```python
from build123d import *

# Parameters (mm, degrees)
F0_R     = 4
F0_R_2   = 5
F1_DEPTH = 8.5


with BuildPart() as f1:
    # F0 (on Top) → F1 (new body, symmetric)
    with BuildSketch(Plane.XY):
        with BuildLine():
            ThreePointArc((175, -20), (195, 0), (175, 20))
            Line((175, 20), (-175, 20))
            ThreePointArc((-175, 20), (-195, 0), (-175, -20))
            Line((-175, -20), (175, -20))
        make_face()
        with Locations((-175, 0)):
            Circle(F0_R, mode=Mode.SUBTRACT)
        Circle(F0_R_2, mode=Mode.SUBTRACT)
        with Locations((175, 0)):
            Circle(F0_R, mode=Mode.SUBTRACT)
    extrude(amount=F1_DEPTH, both=True)


solid = f1.part
```
Geometry: final body of the model. Coordinates: model frame, mm. Round coordinates to 2 decimals unless told otherwise and drop trailing zeros. Write each loop counter-clockwise with the first axis right and the second up, starting at its lowest first coordinate (ties: lowest second). Pieces come first, ordered by that corner, then holes. Notation, with made-up numbers: M 29,15.25 L 71,15.25 A15 cw 71,35.25 Z; hole C -35,61.5 d11. An arc over 180 degrees is marked long. Answer in a Markdown table with one row per item. Add a question column.
(1) Ray query, L1, parallel to Y at x = 175, z = -0.25; L2, parallel to X at y = 3, z = 1.5; L3, parallel to X at y = -1, z = 1.5. Return the intervals inside material, ascending.
(2) Cut plane B-B, the plane z = 5.25. Return the cut outline in (x, y), then the cut area to 3 significant figures.
(3) Cut plane C-C, the plane y = 0. Return the cut outline in (x, z), then the cut area to 3 significant figures.
(4) Cut plane A-A, the plane x = 0. Return the cut outline in (y, z), then the cut area to 3 significant figures.
(5) Draft query along Y for faces 1 (the face through (195, 0, 0)), 2 (the face through (-3, 5, -8.5)), 3 (the face through (178.815, 1.201, -0.119)). Return one class per face: pulls with the +Y half, pulls with the -Y half, needs draft (parallel to the pull), parting line crosses it, or undercut.
(6) Cut plane D-D, the plane y = -15.5. Return the cut outline in (x, z), then the cut area to 3 significant figures.
(7) Contact query for flat-ended pins moving along their axis: pin 1 (5 mm diameter, centred on y = -4, z = -3, fed in from -X); pin 2 (5 mm diameter, centred on y = 1, z = -2, fed in from -X); pin 3 (2 mm diameter, centred on y = -9, z = 3, fed in from -X). Output: stop coordinate, or through.
Established:
| question | item | result |
|---|---|---|
| 1 | L1 | -20 to -4, 4 to 20 |
| 1 | L2 | -194.77 to -177.65, -172.35 to -4, 4 to 172.35, 177.65 to 194.77 |
| 1 | L3 | -194.97 to -178.87, -171.13 to -4.9, 4.9 to 171.13, 178.87 to 194.97 |
| 2 | outline | M -175,-20 L 175,-20 A20 ccw 175,20 L -175,20 A20 ccw Z; hole C -175,0 d8; hole C 0,0 d10; hole C 175,0 d8 |
| 2 | area | 15,100 mm² |
| 3 | outline | M -195,-8.5 L -179,-8.5 L -179,8.5 L -195,8.5 Z; M -171,-8.5 L -5,-8.5 L -5,8.5 L -171,8.5 Z; M 5,-8.5 L 171,-8.5 L 171,8.5 L 5,8.5 Z; M 179,-8.5 L 195,-8.5 L 195,8.5 L 179,8.5 Z |
| 3 | area | 6,190 mm² |
| 4 | outline | M -20,-8.5 L -5,-8.5 L -5,8.5 L -20,8.5 Z; M 5,-8.5 L 20,-8.5 L 20,8.5 L 5,8.5 Z |
| 4 | area | 510 mm² |
| 5 | face 1 | parting line crosses it |
| 5 | face 2 | needs draft |
| 5 | face 3 | undercut |
| 6 | outline | M -187.64,-8.5 L 187.64,-8.5 L 187.64,8.5 L -187.64,8.5 Z |
| 6 | area | 6,380 mm² |
| 7 | pin 1 | x = -194.94 |
| 7 | pin 2 | x = -195 |
| 7 | pin 3 | x = -193.33 |
